from build123d import *

# Parameters (mm, degrees)
SKETCH_1_R      = 5
EXTRUDE_1_DEPTH = 30


with BuildPart() as part:
    # 草圖1 → 填料-伸長1 (new body)
    with BuildSketch(Plane(origin=(0, 0, 0), x_dir=(1, 0, 0), z_dir=(0, 1, 0))):
        with BuildLine():
            Line((24.320676959, 24.968031977), (16.230507016, 30.8458845))
            Line((16.230507016, 30.8458845), (10.352654493, 22.755714556))
            ThreePointArc((10.352654493, 22.755714556), (7.725424859, 23.776412907), (5, 24.494897428))
            Line((5, 24.494897428), (5, 34.494897428))
            Line((5, 34.494897428), (-5, 34.494897428))
            Line((-5, 34.494897428), (-5, 24.494897428))
            ThreePointArc((-5, 24.494897428), (-7.725424859, 23.776412907), (-10.352654493, 22.755714556))
            Line((-10.352654493, 22.755714556), (-16.230507016, 30.8458845))
            Line((-16.230507016, 30.8458845), (-24.320676959, 24.968031977))
            Line((-24.320676959, 24.968031977), (-18.442824436, 16.877862033))
            ThreePointArc((-18.442824436, 16.877862033), (-20.225424859, 14.694631307), (-21.750946843, 12.324622162))
            Line((-21.750946843, 12.324622162), (-31.261512006, 15.414792106))
            Line((-31.261512006, 15.414792106), (-34.35168195, 5.904226943))
            Line((-34.35168195, 5.904226943), (-24.841116787, 2.814056999))
            ThreePointArc((-24.841116787, 2.814056999), (-25, 0), (-24.841116787, -2.814056999))
            Line((-24.841116787, -2.814056999), (-34.35168195, -5.904226943))
            Line((-34.35168195, -5.904226943), (-31.261512006, -15.414792106))
            Line((-31.261512006, -15.414792106), (-21.750946843, -12.324622162))
            ThreePointArc((-21.750946843, -12.324622162), (-20.225424859, -14.694631307), (-18.442824436, -16.877862033))
            Line((-18.442824436, -16.877862033), (-24.320676959, -24.968031977))
            Line((-24.320676959, -24.968031977), (-16.230507016, -30.8458845))
            Line((-16.230507016, -30.8458845), (-10.352654493, -22.755714556))
            ThreePointArc((-10.352654493, -22.755714556), (-7.725424859, -23.776412907), (-5, -24.494897428))
            Line((-5, -24.494897428), (-5, -34.494897428))
            Line((-5, -34.494897428), (5, -34.494897428))
            Line((5, -34.494897428), (5, -24.494897428))
            ThreePointArc((5, -24.494897428), (7.725424859, -23.776412907), (10.352654493, -22.755714556))
            Line((10.352654493, -22.755714556), (16.230507016, -30.8458845))
            Line((16.230507016, -30.8458845), (24.320676959, -24.968031977))
            Line((24.320676959, -24.968031977), (18.442824436, -16.877862033))
            ThreePointArc((18.442824436, -16.877862033), (20.225424859, -14.694631307), (21.750946843, -12.324622162))
            Line((21.750946843, -12.324622162), (31.261512006, -15.414792106))
            Line((31.261512006, -15.414792106), (34.35168195, -5.904226943))
            Line((34.35168195, -5.904226943), (24.841116787, -2.814056999))
            ThreePointArc((24.841116787, -2.814056999), (25, 0), (24.841116787, 2.814056999))
            Line((24.841116787, 2.814056999), (34.35168195, 5.904226943))
            Line((34.35168195, 5.904226943), (31.261512006, 15.414792106))
            Line((31.261512006, 15.414792106), (21.750946843, 12.324622162))
            ThreePointArc((21.750946843, 12.324622162), (20.225424859, 14.694631307), (18.442824436, 16.877862033))
            Line((18.442824436, 16.877862033), (24.320676959, 24.968031977))
        make_face()
        with Locations(Location((0, 0, 0), (0, 0, 270))):
            Circle(SKETCH_1_R, mode=Mode.SUBTRACT)
    extrude(amount=EXTRUDE_1_DEPTH)


solid = part.part
Geometry: final body of the model. Coordinates: model frame, mm. A direction names the side the tool comes from. Give positions to 0.01 mm unless a question says otherwise; leave off trailing zeros. Write each loop counter-clockwise with the first axis right and the second up, starting at its lowest first coordinate (ties: lowest second). Pieces come first, ordered by that corner, then holes. Notation, with made-up numbers: (-34, -15) - (-19, -15) arc R22 cw to (-19, 20) - close; hole circle Ø8 at (64.5, 88.25). An arc over 180 degrees is marked (long way). Return JSON: item names as keys, results as strings. Group by question number.
1) Set-up query: faces 1 (the flat face through (26.44, 14.79, 13.85)), 2 (the flat face through (-20.219, 14.79, -27.948)), 3 (the flat face through (-29.66, 14.79, -4.38)), 4 (the flat face through (13.333, 14.79, -26.857)), 5 (the cylindrical face through (-7.763, 14.79, 23.764)). Return all of +Z, -Z, +X, -X, +Y, -Y with unobstructed straight access to the full face (end or side cutting, diameter ignored); none if empty.
2) First-contact query: P1, Ø2, axis at x = -23.5, z = -14, coming from the -Y side; P2, Ø3, axis at x = -16.5, y = 6, coming from the +Z side; P3, Ø6, axis at x = 23, y = 26.5, coming from the -Z side; P4, Ø5, axis at y = 19.5, z = -29, coming from the -X side. Flat tips, straight axial feed; report the tip coordinate or a pass-through.
3) Section C-C on z = -18.5. Return the cut outline in (x, y).
4) Mould query, pull axis X, two halves, no side actions, for faces 6 (the flat face through (-5, 15, 29)), 7 (the flat face through (-21.423, 14.79, -20.98)), 8 (the flat face through (0, 0, 7)). Classes: released by +X, released by -X, zero draft, split by the parting line, or undercut.
5) Section B-B on z = 0. Return the cut outline in (x, y), plus the area to 3 significant figures.
6) Section D-D on x = -14.5. Return the cut outline in (y, z).
7) Line query: line 1 (X direction, y = 15.5, z = 27.5); line 2 (X direction, y = 10.25, z = 31); line 3 (X direction, y = 25.25, z = 29). Output: solid intervals per line, ascending.
8) Section A-A on x = 0. Return the cut outline in (y, z).
Filled in:
{
 "1": {"face 1": "+Y, -Y", "face 2": "-Z, -X, +Y, -Y", "face 3": "-X, +Y, -Y", "face 4": "-Z, +Y, -Y", "face 5": "+Z, +Y, -Y"},
 "2": {"P1": "passes through", "P2": "stops at z = 30.85", "P3": "stops at z = -28.11", "P4": "stops at x = -22.21"},
 "3": {"outline": "(-19.62, 0) - (19.62, 0) - (19.62, 30) - (-19.62, 30) - close"},
 "4": {"face 6": "undercut", "face 7": "released by -X", "face 8": "zero draft"},
 "5": {"outline": "(-25, 0) - (-5, 0) - (-5, 30) - (-25, 30) - close; (5, 0) - (25, 0) - (25, 30) - (5, 30) - close", "area": "1,200 mm^2"},
 "6": {"outline": "(0, -28.46) - (30, -28.46) - (30, 28.46) - (0, 28.46) - close"},
 "7": {"line 1": "x = -20.84 to -13.8, -5 to 5, 13.8 to 20.84", "line 2": "x = -5 to 5", "line 3": "x = -18.77 to -14.89, -5 to 5, 14.89 to 18.77"},
 "8": {"outline": "(0, -34.49) - (30, -34.49) - (30, -5) - (0, -5) - close; (0, 5) - (30, 5) - (30, 34.49) - (0, 34.49) - close"}
}
